Could you check a few things on this model? Use its own coordinates, in mm. Face numbers are marked on the shaded views. Round coordinates to 2 decimals unless told otherwise and drop trailing zeros. Order: outer loops, then holes, each group sorted by start corner. A loop starts at its lowest first (then second) coordinate and runs counter-clockwise, first axis right, second up.
```python
from build123d import *

# Parameters (mm, degrees)
SKETCH1_R               = 5
SKETCH1_R_2             = 1.75
BOSS_EXTRUDE1_DEPTH     = 33.3
SKETCH2_R               = 2.75
BOSS_EXTRUDE2_DEPTH     = 25.8
BOSS_EXTRUDE3_DEPTH     = 23
SKETCH3_R               = 1.55
CUT_EXTRUDE1_DEPTH      = 3
CUT_EXTRUDE2_DEPTH      = 42.631243075
CUT_EXTRUDE2_DEPTH_BACK = 42.631243075
CHAMFER3_SIZE2          = 2.8
CHAMFER3_SIZE           = 4.849742261


with BuildPart() as part:
    # Sketch1 → Boss-Extrude1 (new body)
    with BuildSketch(Plane(origin=(0, 0, 0), x_dir=(1, 0, 0), z_dir=(0, 1, 0))):
        with Locations(Location((0, 0, 0), (0, 0, 270))):
            Circle(SKETCH1_R)
        with Locations(Location((0, 0, 0), (0, 0, 270))):
            Circle(SKETCH1_R_2, mode=Mode.SUBTRACT)
    extrude(amount=BOSS_EXTRUDE1_DEPTH)



with BuildPart() as body_2:
    # Sketch2 → Boss-Extrude2 (new body)
    with BuildSketch(Plane(origin=(0, 0, 0), x_dir=(1, 0, 0), z_dir=(0, 1, 0))):
        with Locations(Location((21.73, 2, 0), (0, 0, 90))):
            Circle(SKETCH2_R)
    extrude(amount=BOSS_EXTRUDE2_DEPTH)


with BuildPart() as part_1:
    add(part.part)

    add(body_2.part)  # Boss-Extrude3 merges body 2
    # Sketch4 → Boss-Extrude3 (add)
    with BuildSketch(Plane.XZ):
        Polygon((21.637816883, 0.748454524), (0.891372697, 4.919903934), (2.67017604, 0), (0.014392721, -4.999979285), (21.637816883, -4.748454524), align=None)
    extrude(amount=-BOSS_EXTRUDE3_DEPTH)

    # Sketch3 → Cut-Extrude1 (cut)
    with BuildSketch(Plane(origin=(0, 25.8, 0), x_dir=(1, 0, 0), z_dir=(0, 1, 0))):
        with Locations(Location((21.73, 2, 0), (0, 0, 270))):
            Circle(SKETCH3_R)
    extrude(amount=-CUT_EXTRUDE1_DEPTH, mode=Mode.SUBTRACT)

    # Sketch5 → Cut-Extrude2 (cut, two sides: drawn at the far end of the back side and taken through both)
    with BuildSketch(Plane.XY.offset(-CUT_EXTRUDE2_DEPTH_BACK)):
        Polygon((24.48, 23.3), (12.590189784, -2.197780292), (24.48, 0), (24.48, 11.782113075), align=None)
    extrude(amount=CUT_EXTRUDE2_DEPTH + CUT_EXTRUDE2_DEPTH_BACK, mode=Mode.SUBTRACT)

    # Chamfer3
    chamfer3_edges = [part_1.edges().sort_by_distance(p)[0] for p in [
        (18.98, 23, -2),
    ]]
    chamfer3_side = [part_1.faces().sort_by_distance(p)[0] for p in [
        (18.924, 23, -2),
    ]]
    chamfer(chamfer3_edges, length=CHAMFER3_SIZE - 0.0001, length2=CHAMFER3_SIZE2 - 0.0001, reference=chamfer3_side[0])  # a hair under: the kernel refuses the full size


solid = part_1.part
```
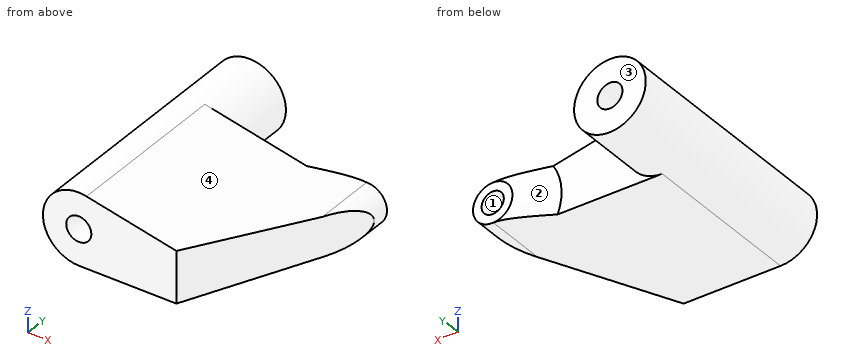
Q1. Imagine slicing it at C-C, the plane y = 14. Please give me the cut outline in (x, z).
Q2. Imagine slicing it at B-B, the plane x = -0.5. Please give me the cut outline in (y, z).
Q3. Imagine slicing it at A-A, the plane y = 24. Please give me the cut outline in (x, z), then the cut area to 3 significant figures.
Q4. I need wall thicknesses on L1, parallel to X at y = 31, z = 0.5; L2, parallel to Y at x = 7.75, z = 1.75; L3, parallel to X at y = 15, z = 0. Which ranges of each line are inside material? Lowest first, please.
Q5. For P1, Ø3, axis at x = 17.5, y = 18, coming from the +Z side; P2, Ø5, axis at y = 17, z = 2, coming from the +X side; P3, Ø3, axis at x = 11, z = 2, coming from the +Y side, each with a flat end and sliding along its axis, tell me the tip position at first contact or that it passes through.
Q6. We'd pull the mould along X, two halves only. Please class the marked faces 1, 2, 3 and 4: released by +X, released by -X, zero draft, split by the parting line, or undercut.
Q7. Imagine slicing it at D-D, the plane z = 2.75. Please give me the cut outline in (x, y), then the cut area to 3 significant figures.
Filled in:
1. outline: (0.1, -5) - (20.14, -4.77) - (20.14, 1.05) - (1.08, 4.88) arc R5 ccw (long way) to start; hole circle Ø3.5 at (0, 0)
2. outline: (0, -4.97) - (33.3, -4.97) - (33.3, -1.68) - (0, -1.68) - close; (0, 1.68) - (33.3, 1.68) - (33.3, 4.97) - (0, 4.97) - close
3. outline: circle Ø10 at (0, 0); (16.58, -4.81) - (21.64, -4.75) arc R2.75 ccw (long way) to (21.64, 0.75) - (17.14, 1.65) arc R5.87 ccw to start; hole circle Ø3.5 at (0, 0); hole circle Ø3.1 at (21.73, -2)
3. area: 107 mm2
4. L1: x = -4.97 to -1.68, 1.68 to 4.97
4. L2: y = 0 to 23
4. L3: x = -5 to -1.75, 1.75 to 20.61
5. P1: stops at z = 1.88
5. P2: stops at x = 22.52
5. P3: stops at y = 23
6. face 1: undercut
6. face 2: undercut
6. face 3: zero draft
6. face 4: released by +X
7. outline: (-4.18, 0) - (11.68, 0) - (11.68, 23) - (4.18, 23) - (4.18, 33.3) - (-4.18, 33.3) - close
7. area: 451 mm2
